Here's how the part is built. I have some questions about the finished solid (model axes, mm). Face numbers are marked on the shaded views. A direction names the side the tool comes from. Round coordinates to 2 decimals unless told otherwise and drop trailing zeros. Write each loop counter-clockwise with the first axis right and the second up, starting at its lowest first coordinate (ties: lowest second). Pieces come first, ordered by that corner, then holes. Notation, with made-up numbers: (49, -20) -> (53, -20) arc R20 ccw to (53, 19) -> close; hole circle Ø11 at (79, -28). An arc over 180 degrees is marked (long way). Answer as CSV lines item,"result".
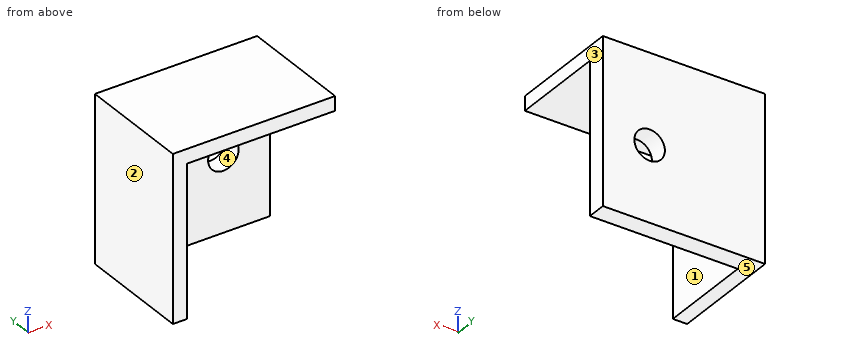
from build123d import *

# Parameters (mm, degrees)
EXTRUDE_1_DEPTH     = 10
SKETCH_2_W          = 17
SKETCH_2_H          = 18.8
SKETCH_2_R          = 1.6
EXTRUDE_2_DEPTH     = 2
SKETCH_4_W          = 17
SKETCH_4_H          = 1.5
CUT_EXTRUDE_1_DEPTH = 29.04353758


with BuildPart() as part:
    # 草图1 → 凸台-拉伸1 (new body)
    with BuildSketch(Plane(origin=(0, 0, 0), x_dir=(1, 0, 0), z_dir=(0, 1, 0))):
        Polygon((1.5, 1.5), (1.5, 17.3), (15.5, 17.3), (17, 17.3), (17, 18.8), (0, 18.8), (0, 0), (17, 0), (17, 1.5), (15.5, 1.5), align=None)
    extrude(amount=EXTRUDE_1_DEPTH)

    # 草图2 → 凸台-拉伸2 (add)
    with BuildSketch(Plane(origin=(0, 10, 0), x_dir=(1, 0, 0), z_dir=(0, 1, 0))):
        with Locations((8.5, 9.4)):
            Rectangle(SKETCH_2_W, SKETCH_2_H)
        with Locations(Location((12.1, 9.4, 0), (0, 0, 270))):
            Circle(SKETCH_2_R, mode=Mode.SUBTRACT)
    extrude(amount=EXTRUDE_2_DEPTH)

    # 草图4 → 切除-拉伸1 (cut, through all)
    with BuildSketch(Plane.XZ):
        with Locations((8.5, -18.05)):
            Rectangle(SKETCH_4_W, SKETCH_4_H)
    extrude(amount=-CUT_EXTRUDE_1_DEPTH, mode=Mode.SUBTRACT)


solid = part.part
Item 1: Suppose I cut it at D-D, the plane y = 4. List the corners of the cut face in (x, z) for me.
Results found:
outline,"(0, -17.3) -> (1.5, -17.3) -> (1.5, -1.5) -> (17, -1.5) -> (17, 0) -> (0, 0) -> close"
Item 2: I need wall thicknesses on L1, parallel to X at y = 11.2, z = -9.4; L2, parallel to Y at x = 7, z = -4; L3, parallel to X at y = 7, z = -2. Which ranges of each line are inside material? Lowest first, please.
Results found:
L1,"x = 0 to 10.5, 13.7 to 17"
L2,"y = 10 to 12"
L3,"x = 0 to 1.5"
Item 3: For the marked faces 1 and 2, which set-ups out of +Z, -Z, +X, -X, +Y, -Y let a thin tool reach every point of the face, with its end or its side?
Results found:
face 1,"-Z, +X, -Y"
face 2,"+Z, -Z, -X, +Y, -Y"
Item 4: Will these pins go through, and if not, where does the flat tip stop? pin 1 (3 mm diameter, centred on x = 12.1, z = -9.4, fed in from -Y); pin 2 (5 mm diameter, centred on y = 3, z = -9, fed in from +X); pin 3 (2 mm diameter, centred on x = 6.5, y = 8.5, fed in from -Z).
Results found:
pin 1,"passes through"
pin 2,"stops at x = 1.5"
pin 3,"stops at z = -1.5"
Item 5: Suppose I cut it at B-B, the plane x = 12.1. List the corners of the cut face in (y, z) for me, then the cut area to 3 significant figures.
Results found:
outline,"(0, -1.5) -> (10, -1.5) -> (10, -7.8) -> (12, -7.8) -> (12, 0) -> (0, 0) -> close; (10, -17.3) -> (12, -17.3) -> (12, -11) -> (10, -11) -> close"
area,"43.2 mm²"
Item 6: Suppose I cut it at C-C, the plane z = -4. List the corners of the cut face in (x, y) for me, then the cut area to 3 significant figures.
Results found:
outline,"(0, 0) -> (1.5, 0) -> (1.5, 10) -> (17, 10) -> (17, 12) -> (0, 12) -> close"
area,"49.0 mm²"
Item 7: Suppose I cut it at A-A, the plane z = -9.4. List the corners of the cut face in (x, y) for me, then the cut area to 3 significant figures.
Results found:
outline,"(0, 0) -> (1.5, 0) -> (1.5, 10) -> (10.5, 10) -> (10.5, 12) -> (0, 12) -> close; (13.7, 10) -> (17, 10) -> (17, 12) -> (13.7, 12) -> close"
area,"42.6 mm²"
Item 8: If we mould it in two halves opening along X, with no side actions, what happens to the marked faces 3, 4 and 5? For each: pulls with the +X half, pulls with the -X half, needs draft (parallel to the pull), parting line crosses it, or undercut.
Results found:
face 3,"pulls with the +X half"
face 4,"undercut"
face 5,"needs draft"
